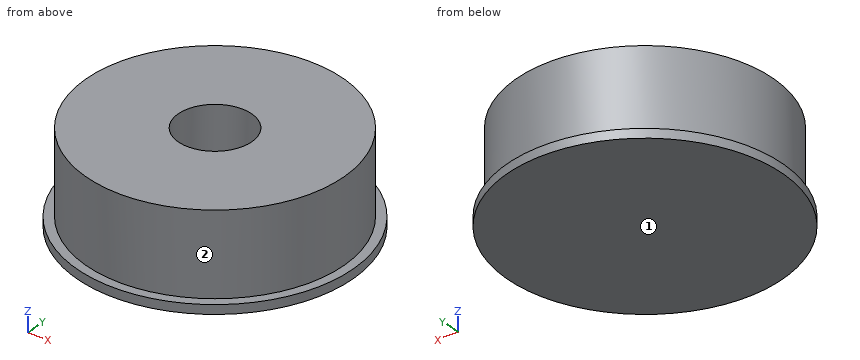
```python
from build123d import *

# Parameters (mm, degrees)
SKETCH1_R           = 87.5
SKETCH1_R_2         = 25
BOSS_EXTRUDE1_DEPTH = 62.5
SKETCH2_R           = 93.75
BOSS_EXTRUDE3_DEPTH = 6.25


with BuildPart() as part:
    # Sketch1 → Boss-Extrude1 (new body)
    with BuildSketch(Plane.XY):
        Circle(SKETCH1_R)
        Circle(SKETCH1_R_2, mode=Mode.SUBTRACT)
    extrude(amount=BOSS_EXTRUDE1_DEPTH)

    # Sketch2 → Boss-Extrude3 (add)
    with BuildSketch(Plane.XY):
        Circle(SKETCH2_R)
    extrude(amount=BOSS_EXTRUDE3_DEPTH)


solid = part.part
```
Here's how the part is built. I have some questions about the finished solid (model axes, mm). Face numbers are marked on the shaded views. A direction names the side the tool comes from. Give positions to 0.01 mm unless a question says otherwise; leave off trailing zeros. Loops run counter-clockwise (first coordinate to the right, second up) from the corner with the lowest first, then second, coordinate; pieces in that order, holes last. Notation, with made-up numbers: M 43,70.25 L 99,70.25 A27 ccw 99,93.25 Z; hole C -21,34.5 d11. An arc over 180 degrees is marked long. Put each result on its own line as item: value. Start each with the question number.
(1) For the marked faces 1 and 2, which set-ups out of +Z, -Z, +X, -X, +Y, -Y let a thin tool reach every point of the face, with its end or its side?
(2) I want a section at D-D on x = 30. Please give me the cut outline in (y, z).
(3) Will these pins go through, and if not, where does the flat tip stop? pin 1 Ø15 at (x, y) = (2.5, -2.5) entering from +Z; pin 2 Ø4 at (y, z) = (19, 37) entering from +X; pin 3 Ø12 at (y, z) = (-23, 9) entering from +X.
(4) I need wall thicknesses on line 1 along Y through (x, z) = (0, 25); line 2 along Z through (x, y) = (-19.5, 8). Which ranges of each line are inside material? Lowest first, please. Write a range as [from, to].
(5) I want a section at C-C on z = 14. Please give me the cut outline in (x, y), then the cut area to 3 significant figures.
(6) I want a section at A-A on y = 0. Please give me the cut outline in (x, z), then the cut area to 3 significant figures.
Answer block:
1. face 1: -Z, +X, -X, +Y, -Y
1. face 2: +Z
2. outline: M -88.82,0 L 88.82,0 L 88.82,6.25 L 82.2,6.25 L 82.2,62.5 L -82.2,62.5 L -82.2,6.25 L -88.82,6.25 Z
3. pin 1: z = 6.25
3. pin 2: x = 85.83
3. pin 3: x = 92.07
4. line 1: [-87.5, -25], [25, 87.5]
4. line 2: [0, 6.25]
5. outline: C 0,0 d175; hole C 0,0 d50
5. area: 22,100 mm^2
6. outline: M -93.75,0 L 93.75,0 L 93.75,6.25 L 87.5,6.25 L 87.5,62.5 L 25,62.5 L 25,6.25 L -25,6.25 L -25,62.5 L -87.5,62.5 L -87.5,6.25 L -93.75,6.25 Z
6. area: 8,200 mm^2
